Can you work these out from the model? Positions are in its coordinate system, mm. Face numbers are marked on the shaded views. A direction names the side the tool comes from. Round coordinates to 2 decimals unless told otherwise and drop trailing zeros. Loops run counter-clockwise (first coordinate to the right, second up) from the corner with the lowest first, then second, coordinate; pieces in that order, holes last.
from build123d import *

# Parameters (mm, degrees)
SKETCH1_W           = 30
SKETCH1_H           = 23
BOSS_EXTRUDE1_DEPTH = 25
SKETCH2_R           = 8
CUT_EXTRUDE1_DEPTH  = 5
SKETCH3_R           = 7
CUT_EXTRUDE2_DEPTH  = 1
SKETCH4_R           = 1.9
CUT_EXTRUDE3_DEPTH  = 4
SKETCH6_R           = 9
CUT_EXTRUDE4_DEPTH  = 4
SKETCH7_R           = 3
CUT_EXTRUDE8_DEPTH  = 19
SKETCH12_R          = 8
CUT_EXTRUDE9_DEPTH  = 1
CHAMFER1_SIZE       = 2.5
CHAMFER2_SIZE       = 0.5


with BuildPart() as part:
    # Sketch1 → Boss-Extrude1 (new body)
    with BuildSketch(Plane(origin=(0, 0, 0), x_dir=(1, 0, 0), z_dir=(0, 1, 0))):
        with Locations((15, 1)):
            Rectangle(SKETCH1_W, SKETCH1_H)
    extrude(amount=BOSS_EXTRUDE1_DEPTH)

    # Sketch2 → Cut-Extrude1 (cut)
    with BuildSketch(Plane(origin=(30, 0, 0), x_dir=(0, 0, -1), z_dir=(1, 0, 0))):
        with Locations((1, 12.5)):
            Circle(SKETCH2_R)
    cut_extrude1 = extrude(amount=-CUT_EXTRUDE1_DEPTH, mode=Mode.SUBTRACT)

    # Sketch3 → Cut-Extrude2 (cut)
    with BuildSketch(Plane(origin=(25, 0, 0), x_dir=(0, 0, -1), z_dir=(1, 0, 0))):
        with Locations((1, 12.5)):
            Circle(SKETCH3_R)
    cut_extrude2 = extrude(amount=-CUT_EXTRUDE2_DEPTH, mode=Mode.SUBTRACT)

    # Sketch4 → Cut-Extrude3 (cut)
    with BuildSketch(Plane(origin=(24, 0, 0), x_dir=(0, 0, -1), z_dir=(1, 0, 0))):
        with Locations((1, 12.5)):
            Circle(SKETCH4_R)
    cut_extrude3 = extrude(amount=-CUT_EXTRUDE3_DEPTH, mode=Mode.SUBTRACT)

    # Mirror1: Cut-Extrude1, Cut-Extrude2, Cut-Extrude3 across plane
    add(cut_extrude1.mirror(Plane(origin=(15, 25, 0), x_dir=(0, 0, 1), z_dir=(1, 0, 0))), mode=Mode.SUBTRACT)
    add(cut_extrude2.mirror(Plane(origin=(15, 25, 0), x_dir=(0, 0, 1), z_dir=(1, 0, 0))), mode=Mode.SUBTRACT)
    add(cut_extrude3.mirror(Plane(origin=(15, 25, 0), x_dir=(0, 0, 1), z_dir=(1, 0, 0))), mode=Mode.SUBTRACT)

    # Sketch6 → Cut-Extrude4 (cut)
    with BuildSketch(Plane.XY.offset(10.5)):
        with Locations((15, 12.5)):
            Circle(SKETCH6_R)
    cut_extrude4 = extrude(amount=-CUT_EXTRUDE4_DEPTH, mode=Mode.SUBTRACT)

    # Sketch7 → Cut-Extrude8 (cut)
    with BuildSketch(Plane.XY.offset(6.5)):
        with Locations((15, 12.5)):
            Circle(SKETCH7_R)
    extrude(amount=-CUT_EXTRUDE8_DEPTH, mode=Mode.SUBTRACT)

    # Sketch12 → Cut-Extrude9 (cut)
    with BuildSketch(Plane.XY.offset(6.5)):
        with Locations((15, 12.5)):
            Circle(SKETCH12_R)
    cut_extrude9 = extrude(amount=-CUT_EXTRUDE9_DEPTH, mode=Mode.SUBTRACT)

    # Mirror4: Cut-Extrude4, Cut-Extrude9 across plane
    add(cut_extrude4.mirror(Plane(origin=(15, 0, -1), x_dir=(1, 0, 0), z_dir=(0, 0, 1))), mode=Mode.SUBTRACT)
    add(cut_extrude9.mirror(Plane(origin=(15, 0, -1), x_dir=(1, 0, 0), z_dir=(0, 0, 1))), mode=Mode.SUBTRACT)

    # Chamfer1
    chamfer1_edges = [part.edges().sort_by_distance(p)[0] for p in [
        (15, 25, -12.5),
        (15, 0, -12.5),
        (15, 0, 10.5),
        (15, 25, 10.5),
    ]]
    chamfer(chamfer1_edges, length=CHAMFER1_SIZE)

    # Chamfer2
    chamfer2_edges = [part.edges().sort_by_distance(p)[0] for p in [
        (30, 12.5, 7),
        (0, 12.5, 7),
        (6, 12.5, 10.5),
        (6, 12.5, -12.5),
    ]]
    chamfer(chamfer2_edges, length=CHAMFER2_SIZE)


solid = part.part
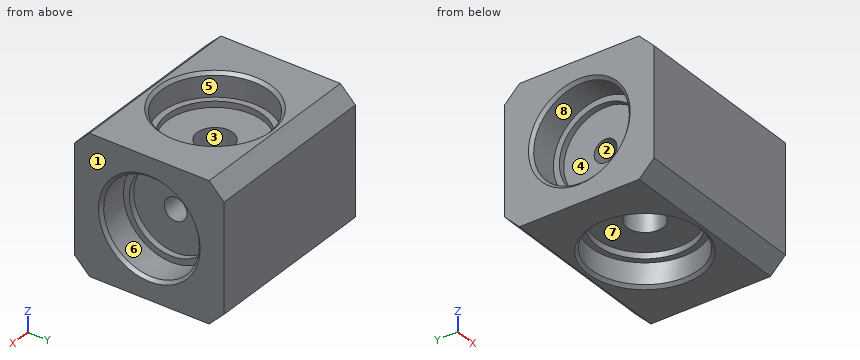
(1) For the marked faces 5, 6, 7 and 8, which set-ups out of +Z, -Z, +X, -X, +Y, -Y let a thin tool reach every point of the face, with its end or its side?
Worked answers:
face 5: +Z
face 6: +X
face 7: -Z
face 8: -X
(2) Will these pins go through, and if not, where does the flat tip stop? P1, Ø7, axis at x = 15, y = 12.5, coming from the +Z side; P2, Ø6, axis at y = 9.5, z = -1, coming from the +X side; P3, Ø9, axis at x = 18.5, y = 11, coming from the +Z side.
Worked answers:
P1: stops at z = 5.5
P2: stops at x = 24
P3: stops at z = 6.5
(3) If we section it at C-C, the plane y = 23.5: List the corners of the cut face in (x, z) for me, then the cut area to 3 significant figures.
Worked answers:
outline: (0, -11.5) - (30, -11.5) - (30, 9.5) - (0, 9.5) - close
area: 630 mm2
(4) If we mould it in two halves opening along X, with no side actions, what happens to the marked faces 1, 2, 3 and 4? For each: released by +X, released by -X, zero draft, split by the parting line, or undercut.
Worked answers:
face 1: released by +X
face 2: zero draft
face 3: undercut
face 4: released by -X
(5) If I drill on line 1 (Y direction, x = 15, z = -3); line 2 (Y direction, x = 27.35, z = -1); line 3 (X direction, y = 17.5, z = -3.25), over which ranges is the centre line in solid material (lowest first)?
Worked answers:
line 1: y = 0 to 9.5, 15.5 to 25
line 2: y = 0 to 4.5, 20.5 to 25
line 3: x = 6 to 24
